Geometry: final body of the model. Coordinates: model frame, mm. A direction names the side the tool comes from. Round coordinates to 2 decimals unless told otherwise and drop trailing zeros. Loops run counter-clockwise (first coordinate to the right, second up) from the corner with the lowest first, then second, coordinate; pieces in that order, holes last. Notation, with made-up numbers: (-38, -32) - (-18, -32) arc R26 ccw to (-18, -9) - close; hole circle Ø2 at (12, -24). An arc over 180 degrees is marked (long way). Answer as a JSON object with one key per item and string values. Group by question number.
Item 1: Draft query along Z for faces 6 (the face through (1, 2, 0)), 7 (the face through (35, 1, -25)), 8 (the face through (35, 1, 25)). Return one class per face: released by +Z, released by -Z, zero draft, split by the parting line, or undercut.
Item 2: Section C-C (x = -19). Return the cut outline in (y, z), plus the area to 3 significant figures.
Item 3: First-contact query: pin 1 (1 mm diameter, centred on x = 2, y = 2, fed in from -Z); pin 2 (1 mm diameter, centred on x = 35, y = 0.5, fed in from +Z); pin 3 (1 mm diameter, centred on x = -13, y = 0.5, fed in from +Z). Flat tips, straight axial feed; report the tip coordinate or a pass-through.
Item 4: Section A-A (x = 24.5). Return the cut outline in (y, z), plus the area to 3 significant figures.
Item 5: Section D-D (z = -32). Return the cut outline in (x, y), plus the area to 3 significant figures.
Item 6: Line query: line 1 (X direction, y = 0.5, z = 9); line 2 (Z direction, x = 24.5, y = 0.9); line 3 (Z direction, x = 8.5, y = 1.7). Output: solid intervals per line, ascending.
Item 7: Section B-B (z = 11). Return the cut outline in (x, y).
Item 8: Reachability of faces 1 (the face through (4, 1, 35.5)), 2 (the face through (-33, 1, -12.5)), 3 (the face through (21, 1, 37)), 4 (the face through (-21, 1, -39)), 5 (the face through (35, 1, 0)) from +Z, -Z, +X, -X, +Y, -Y: full face, straight path, thin tool, end or side. Return the list, or none.
Autodesk Inventor part; units mm, degrees
ref_plane "YZ Plane" through (0, 0, 0) normal (1, 0, 0) x (0, 1, 0)
ref_plane "XZ Plane" through (0, 0, 0) normal (0, 1, 0) x (-1, 0, 0)
ref_plane "XY Plane" through (0, 0, 0) normal (0, 0, 1) x (1, 0, 0)
sketch "Sketch1" plane through (0, 0, 0) normal (0, 1, 0) x (-1, 0, 0)
  line L0 (34, 37.5) -> (-34, -37.5) construction
  line L1 (-34, 37.5) -> (34, -37.5) construction
  line L2 (34, 37.5) -> (34, 25)
  line L3 (34, 25) -> (32, 25)
  line L4 (32, 25) -> (32, 12.5)
  line L5 (32, 12.5) -> (34, 12.5)
  line L6 (34, 12.5) -> (34, 0)
  line L7 (34, 0) -> (32, 0)
  line L8 (32, 0) -> (32, -12.5)
  line L9 (32, -12.5) -> (34, -12.5)
  line L10 (34, -12.5) -> (34, -25)
  line L11 (34, -25) -> (32, -25)
  line L12 (32, -25) -> (32, -37.5)
  line L13 (34, -25) -> (34, -12.5)
  line L14 (34, 0) -> (34, 12.5)
  line L15 (34, 25) -> (34, 37.5)
  line L16 (32, -39.5) -> (21, -39.5)
  line L17 (21, -39.5) -> (21, -37.5)
  line L18 (21, -37.5) -> (10, -37.5)
  line L19 (10, -37.5) -> (10, -39.5)
  line L20 (10, -39.5) -> (-1, -39.5)
  line L21 (-1, -39.5) -> (-1, -37.5)
  line L22 (-1, -37.5) -> (-12, -37.5)
  line L23 (-12, -37.5) -> (-12, -39.5)
  line L24 (-12, -39.5) -> (-23, -39.5)
  line L25 (-36, -37.5) -> (-36, -25)
  line L26 (-36, -25) -> (-34, -25)
  line L27 (-34, -25) -> (-34, -12.5)
  line L28 (-34, -12.5) -> (-36, -12.5)
  line L29 (-36, -12.5) -> (-36, 0)
  line L30 (-36, 0) -> (-34, 0)
  line L31 (-34, 0) -> (-34, 12.5)
  line L32 (-34, 12.5) -> (-34, 8.9552)
  line L33 (-34, 12.5) -> (-36, 12.5)
  line L34 (-36, 12.5) -> (-36, 25)
  line L35 (-36, 25) -> (-34, 25)
  line L36 (10, -37.5) -> (21, -37.5)
  line L37 (-34, -37.5) -> (-24.5, -37.5)
  line L38 (-12, -37.5) -> (-1, -37.5)
  line L39 (-34, -12.5) -> (-34, -25)
  line L40 (-34, 35.5) -> (-34, 25)
  line L41 (-34, 12.5) -> (-34, 0)
  line L42 (34, 37.5) -> (23, 37.5)
  line L43 (23, 37.5) -> (23, 35.5)
  line L44 (23, 35.5) -> (12, 35.5)
  line L45 (12, 35.5) -> (12, 37.5)
  line L46 (12, 37.5) -> (1, 37.5)
  line L47 (1, 37.5) -> (1, 35.5)
  line L48 (1, 35.5) -> (-10, 35.5)
  line L49 (-10, 35.5) -> (-10, 37.5)
  line L50 (-10, 37.5) -> (-21, 37.5)
  line L51 (-21, 37.5) -> (-21, 35.5)
  line L52 (-21, 35.5) -> (-34, 35.5)
  line L53 (34, 37.5) -> (23, 37.5)
  line L54 (12, 37.5) -> (1, 37.5)
  line L55 (-10, 37.5) -> (-21, 37.5)
  line L56 (-26, 12.25) -> (-19, 12.25)
  line L57 (-19, 12.25) -> (-19, 0.25)
  line L58 (-19, 0.25) -> (-26, 0.25)
  line L59 (-26, 0.25) -> (-26, 12.25)
  line L60 (-26, 12.25) -> (-19, 0.25) construction
  line L61 (-19, 12.25) -> (-26, 0.25) construction
  line L62 (32, -37.5) -> (34, -37.5)
  line L63 (34, -39.5) -> (32, -39.5)
  line L64 (34, -37.5) -> (34, -39.5)
  line L65 (-34, -37.5) -> (-36, -37.5)
  line L66 (-23, -39.5) -> (-23, -37.5)
  line L67 (-23, -37.5) -> (-24.5, -37.5)
  point P0 (0, 0)
  point P1 (-35.8133, -39.5)
  dimension "d3" = 2
  dimension "d4" = 12.5
  dimension "d5" = 12.5
  dimension "d6" = 12.5
  dimension "d7" = 12.5
  dimension "d11" = 11
  dimension "d12" = 11
  dimension "d13" = 11
  dimension "d14" = 11
  dimension "d17" = 12.5
  dimension "d18" = 2
  dimension "d19" = 12.5
  dimension "d20" = 12.5
  dimension "d21" = 2
  dimension "d22" = 12.5
  dimension "d23" = 11
  dimension "d26" = 11
  dimension "d28" = 11
  dimension "d29" = 11
  dimension "d32" = 7
  dimension "d33" = 12
  dimension "d36" = 13
extrude "Extrusion1" add sketch "Sketch1" along normal blind 2
properties part number "KANAN"
Values:
{
 "1": {"face 6": "zero draft", "face 7": "undercut", "face 8": "released by +Z"},
 "2": {"outline": "(0, -37.5) - (2, -37.5) - (2, 35.5) - (0, 35.5) - close", "area": "146 mm^2"},
 "3": {"pin 1": "stops at z = -37.5", "pin 2": "stops at z = 25", "pin 3": "stops at z = 35.5"},
 "4": {"outline": "(0, -37.5) - (2, -37.5) - (2, 0.25) - (0, 0.25) - close; (0, 12.25) - (2, 12.25) - (2, 35.5) - (0, 35.5) - close", "area": "122 mm^2"},
 "5": {"outline": "(-32, 0) - (36, 0) - (36, 2) - (-32, 2) - close", "area": "136 mm^2"},
 "6": {"line 1": "x = -34 to 19, 26 to 34", "line 2": "z = -37.5 to 0.25, 12.25 to 35.5", "line 3": "z = -37.5 to 35.5"},
 "7": {"outline": "(-34, 0) - (19, 0) - (19, 2) - (-34, 2) - close; (26, 0) - (34, 0) - (34, 2) - (26, 2) - close"},
 "8": {"face 1": "+Z, +Y, -Y", "face 2": "-X, +Y, -Y", "face 3": "+Z, +X, +Y, -Y", "face 4": "-Z, +Y, -Y", "face 5": "+X, +Y, -Y"}
}
